CAD build for the part. Positions are in the model's coordinates, mm. Face numbers are marked on the shaded views. A direction names the side the tool comes from. Give positions to 0.01 mm unless a question says otherwise; leave off trailing zeros. Loops run counter-clockwise (first coordinate to the right, second up) from the corner with the lowest first, then second, coordinate; pieces in that order, holes last.
Item 1: Probe probe 1 along X at (y, z) = (-198.5, 73.5); probe 2 along Z at (x, y) = (-25.5, -112.5) (3 decimals); probe 3 along X at (y, z) = (-182, 67.5). List the from-to ranges inside material, lowest first.
Item 2: Drop flat-ended pins along their axis: P1, Ø4, axis at x = -69, y = -121, coming from the -Z side; P2, Ø6, axis at y = -58.5, z = 39.5, coming from the -X side; P3, Ø8, axis at y = -213, z = 49.5, coming from the +X side. Give the stop position or say it passes through.
Item 3: Saw through at D-D on y = -116. Give the cut face in (x, z).
Item 4: Saw through at A-A on y = -152.4. Give the cut face in (x, z), plus the area to 3 significant figures.
Item 5: Mould opens along Y. For the marked faces 4, 5 and 6 say: released by +Y, released by -Y, zero draft, split by the parting line, or undercut.
Item 6: Which spindle directions (+Z, -Z, +X, -X, +Y, -Y) get a long thin tool onto all of the face, cutting with end or side? Do the marked faces 1, 2 and 3. Say none if no direction does.
Item 7: Saw through at C-C on x = -30. Give the cut face in (y, z).
Item 8: Saw through at B-B on z = 56.5. Give the cut face in (x, y).
from build123d import *

# Parameters (mm, degrees)
F0_W      = 152.4
F0_H      = 76.2
F1_DEPTH  = 304.8
F3_DEPTH  = 304.8
F5_DEPTH  = 304.8
F7_DEPTH  = 304.8
F9_DEPTH  = 304.8
F11_DEPTH = 304.8
F13_DEPTH = 304.8
F15_DEPTH = 304.8
F16_R     = 50.8
F17_DEPTH = 22.86


with BuildPart() as f1:
    # F0 (on Front) → F1 (new body)
    with BuildSketch(Plane.XZ):
        with Locations((-76.2, 38.1)):
            Rectangle(F0_W, F0_H)
    extrude(amount=F1_DEPTH)

    # F2 (on Right) → F3 (cut)
    with BuildSketch(Plane.YZ):
        Polygon((-304.8, 0), (0, 0), (-304.8, 76.2), align=None)
    extrude(amount=-F3_DEPTH, mode=Mode.SUBTRACT)

    # F4 (on Front) → F5 (cut)
    with BuildSketch(Plane.XZ):
        Polygon((-38.1, 0), (0, 0), (0, 76.2), align=None)
    extrude(amount=F5_DEPTH, mode=Mode.SUBTRACT)

    # F6 (on Front) → F7 (cut)
    with BuildSketch(Plane.XZ):
        Polygon((-152.4, 0), (-114.3, 0), (-152.4, 76.2), align=None)
    extrude(amount=F7_DEPTH, mode=Mode.SUBTRACT)

    # F8 (on Right) → F9 (cut)
    with BuildSketch(Plane.YZ):
        Polygon((-304.8, 76.2), (-304.8, 55.721472), (-289.56, 76.2), align=None)
    extrude(amount=-F9_DEPTH, mode=Mode.SUBTRACT)

    # F10 (on Front) → F11 (cut)
    with BuildSketch(Plane.XZ):
        Polygon((-12.7, 76.2), (0, 38.1), (0, 76.2), align=None)
    extrude(amount=F11_DEPTH, mode=Mode.SUBTRACT)

    # F12 (on Front) → F13 (cut)
    with BuildSketch(Plane.XZ):
        Polygon((-152.4, 76.2), (-152.4, 38.1), (-139.7, 76.2), align=None)
    extrude(amount=F13_DEPTH, mode=Mode.SUBTRACT)

    # F14 (on Front) → F15 (cut)
    with BuildSketch(Plane.XZ):
        Polygon((-76.2, 0), (-38.1, 0), (-76.2, 25.4), align=None)
        Polygon((-114.3, 0), (-76.2, 0), (-76.2, 25.4), align=None)
    extrude(amount=F15_DEPTH, mode=Mode.SUBTRACT)

    # F16 (on face) → F17 (cut)
    with BuildSketch(Plane.XY.offset(76.2)):
        with Locations((-76.2, -152.4)):
            Circle(F16_R)
    extrude(amount=-F17_DEPTH, mode=Mode.SUBTRACT)


solid = f1.part
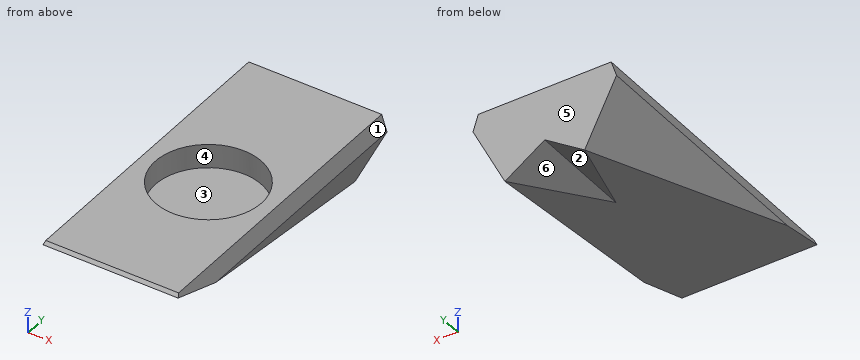
Results below:
1. probe 1: x = -140.6 to -97.54, -54.86 to -11.8
1. probe 2: z = 28.125 to 76.2
1. probe 3: x = -142.6 to -117.49, -34.91 to -9.8
2. P1: stops at z = 29.75
2. P2: stops at x = -135.55
2. P3: stops at x = -11.35
3. outline: (-144.78, 60.96) - (-128.8, 29) - (-23.6, 29) - (-7.62, 60.96) - (-12.7, 76.2) - (-40.76, 76.2) - (-40.76, 53.34) - (-111.64, 53.34) - (-111.64, 76.2) - (-139.7, 76.2) - close
4. outline: (-144.78, 60.96) - (-133.35, 38.1) - (-19.05, 38.1) - (-7.62, 60.96) - (-12.7, 76.2) - (-25.4, 76.2) - (-25.4, 53.34) - (-127, 53.34) - (-127, 76.2) - (-139.7, 76.2) - close
4. area: 2,560 mm2
5. face 4: undercut
5. face 5: released by +Y
5. face 6: zero draft
6. face 1: +Z, +X, +Y, -Y
6. face 2: -Z, +Y, -Y
6. face 3: +Z
7. outline: (-291.95, 72.99) - (-64.8, 16.2) - (0, 16.2) - (0, 76.2) - (-131.28, 76.2) - (-131.28, 53.34) - (-173.52, 53.34) - (-173.52, 76.2) - (-289.56, 76.2) - close
8. outline: (-142.55, -226) - (-9.85, -226) - (-9.85, 0) - (-142.55, 0) - close; hole circle Ø101.6 at (-76.2, -152.4)
